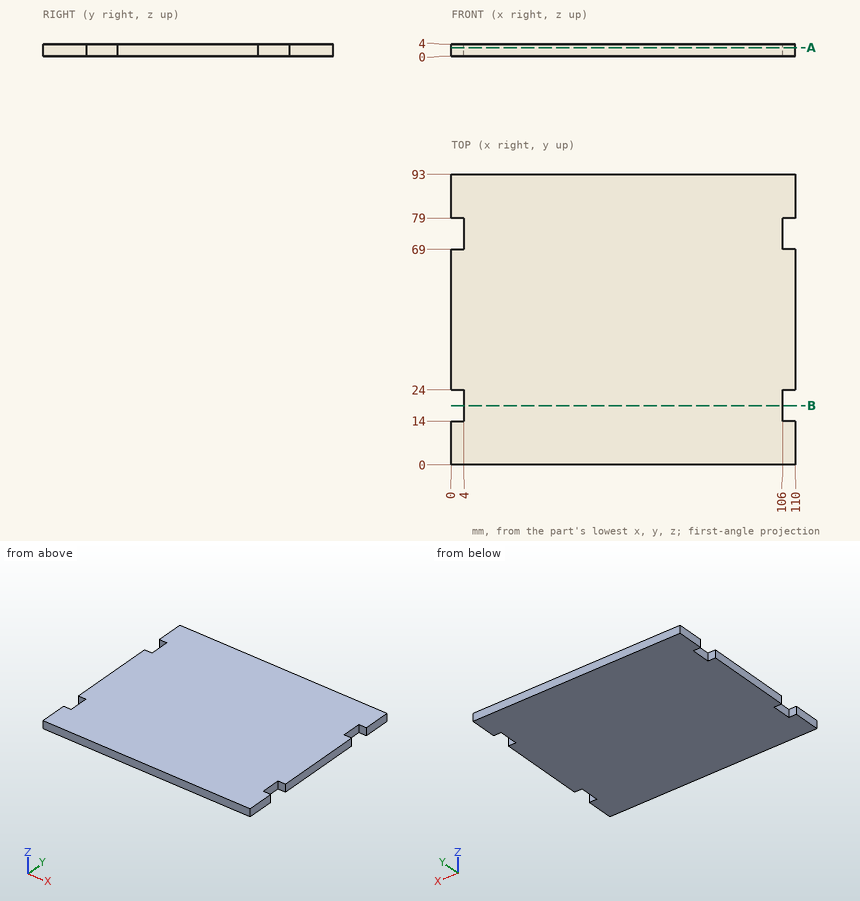
Geometry check sheet. Reference: drawing and pictorial views, mm from the part's lowest x, y, z. Give positions to 0.01 mm unless a question says otherwise; leave off trailing zeros. Order: outer loops, then holes, each group sorted by start corner. A loop starts at its lowest first (then second) coordinate and runs counter-clockwise, first axis right, second up. Notation, with made-up numbers: M -39.5,8.5 L 13.5,8.5 A24 ccw 13.5,38.5 Z; hole C 42.5,33 d4. An arc over 180 degrees is marked long. Answer as a JSON object with one key per item and string values. Group by question number.
1) Scan line: line 1 along X through (y, z) = (17, 0.4). Record every from-to range of solid material in increasing order. Write a range as [from, to].
2) Cross-section at B-B (y = 19). Enter the section's corners in (x, z), then the cut area to 3 significant figures.
3) Depth check by flat-ended pin: pin 1 Ø2 at (y, z) = (73, 1.5) entering from +X; pin 2 Ø2 at (y, z) = (17, 3) entering from -X. Enter the tip coordinate at first touch or a pass-through.
4) Cross-section at A-A (z = 2.8). Enter the section's corners in (x, y).
Result sheet:
{
 "1": {"line 1": "x = [4, 106]"},
 "2": {"outline": "M 4,0 L 106,0 L 106,4 L 4,4 Z", "area": "408 mm2"},
 "3": {"pin 1": "stops at x = 106", "pin 2": "stops at x = 4"},
 "4": {"outline": "M 0,0 L 110,0 L 110,14 L 106,14 L 106,24 L 110,24 L 110,69 L 106,69 L 106,79 L 110,79 L 110,93 L 0,93 L 0,79 L 4,79 L 4,69 L 0,69 L 0,24 L 4,24 L 4,14 L 0,14 Z"}
}
